Here's the drawing with two shaded views (mm, measured from the low corner). I have some questions. A direction names the side the tool comes from. Round coordinates to 2 decimals unless told otherwise and drop trailing zeros. Write each loop counter-clockwise with the first axis right and the second up, starting at its lowest first coordinate (ties: lowest second). Pieces come first, ordered by that corner, then holes. Notation, with made-up numbers: M -9,15 L 27,15 A14 ccw 27,20 Z; hole C -10.75,46.25 d8. An arc over 180 degrees is marked long. Answer as a JSON object with one key per item and string values. Group by question number.
1) Suppose I cut it at D-D, the plane x = 10. Write out the boundary of the cut face in (y, z).
2) Please list where these lines run through material, in increasing order: L1, parallel to X at y = 7, z = 6; L2, parallel to Z at x = 2.75, y = 2.75; L3, parallel to Y at x = 11, z = 1.5. Write a range as [from, to].
3) On a 3-axis mill with a long thin cutter (end or side, diameter ignored), from which of +Z, -Z, +X, -X, +Y, -Y can I reach the whole of each face in a straight line? I mean the marked faces 4, 5, 6, 7 and 8. Say none if no direction works.
4) I'm going to push flat-ended pins straight in: pin 1 Ø2.5 at (y, z) = (5.5, 3) entering from +X; pin 2 Ø6 at (x, z) = (11, 1.5) entering from -Y; pin 3 Ø2 at (x, y) = (10.5, 4.5) entering from -Z; pin 4 Ø0.6 at (y, z) = (9, 10.5) entering from +X. Where does each tip first touch, or does it pass through?
5) If we mould it in two halves opening along X, with no side actions, what happens to the marked faces 1, 2 and 3? For each: +X half, -X half, draft (parallel to the pull), parting line (faces both ways), or undercut.
6) Suppose I cut it at B-B, the plane z = 3.5. Write out the boundary of the cut face in (x, y).
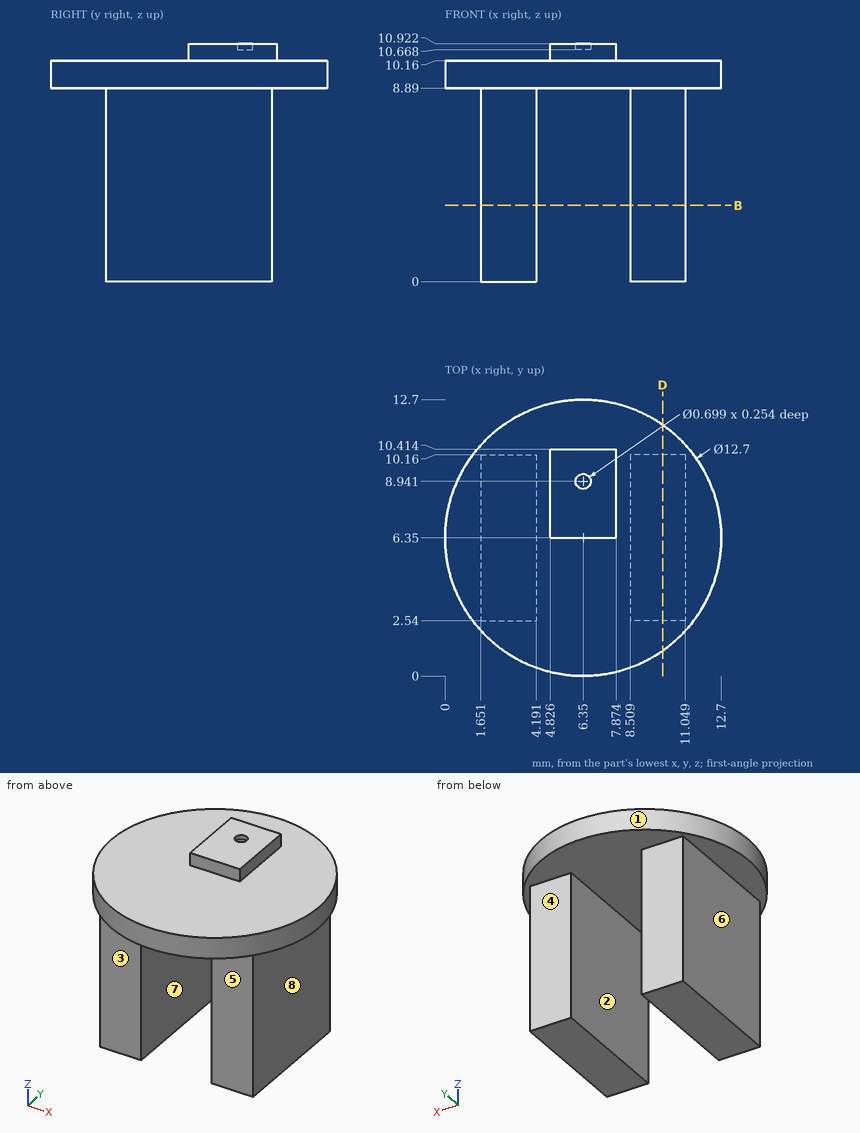
Results:
{
 "1": {"outline": "M 1.15,8.89 L 2.54,8.89 L 2.54,0 L 10.16,0 L 10.16,8.89 L 11.55,8.89 L 11.55,10.16 L 1.15,10.16 Z"},
 "2": {"L1": "[1.65, 4.19], [8.51, 11.05]", "L2": "[0, 10.16]", "L3": "[2.54, 10.16]"},
 "3": {"face 4": "-Z, +X, -X, +Y", "face 5": "-Z, +X, -X, -Y", "face 6": "-Z, -X, +Y, -Y", "face 7": "-Z, +Y, -Y", "face 8": "-Z, +X, +Y, -Y"},
 "4": {"pin 1": "x = 11.05", "pin 2": "y = 2.54", "pin 3": "z = 0", "pin 4": "x = 7.87"},
 "5": {"face 1": "parting line", "face 2": "undercut", "face 3": "draft"},
 "6": {"outline": "M 1.65,2.54 L 4.19,2.54 L 4.19,10.16 L 1.65,10.16 Z; M 8.51,2.54 L 11.05,2.54 L 11.05,10.16 L 8.51,10.16 Z"}
}
